from build123d import *

# Parameters (mm, degrees)
SKETCH_3_R = 1.1


with BuildPart() as part:
    # 扫描1: sweep along a path in 草图1
    with BuildLine(Plane.XY) as sweep_1_path:
        Line((2.063476324, 0), (13.736523676, 0))
        ThreePointArc((13.736523676, 0), (15.17265372, 0.608047955), (15.735547828, 2.062469505))
        Line((15.735547828, 2.062469505), (15.343889389, 14.595539539))
        ThreePointArc((15.343889389, 14.595539539), (14.923518493, 15.761017061), (13.897319856, 16.455254701))
        ThreePointArc((13.897319856, 16.455254701), (7.9, 17.3), (1.902680144, 16.455254701))
        ThreePointArc((1.902680144, 16.455254701), (0.876481507, 15.761017061), (0.456110611, 14.595539539))
        Line((0.456110611, 14.595539539), (0.064452172, 2.062469505))
        ThreePointArc((0.064452172, 2.062469505), (0.62734628, 0.608047955), (2.063476324, 0))
    # 草图3 → 扫描1 (sweep)
    with BuildSketch(Plane(origin=(7.6, 0, 0), x_dir=(0, 0, -1), z_dir=(1, 0, 0))):
        Circle(SKETCH_3_R)
    sweep(path=sweep_1_path.line)


solid = part.part
Can you work these out from the model? Positions are in its coordinate system, mm. Give positions to 0.01 mm unless a question says otherwise; leave off trailing zeros. Order: outer loops, then holes, each group sorted by start corner. A loop starts at its lowest first (then second) coordinate and runs counter-clockwise, first axis right, second up. Notation, with made-up numbers: (2.25, 47) - (13.25, 47) arc R22 ccw to (13.25, 69) - close; hole circle Ø9 at (67, 32). An arc over 180 degrees is marked (long way). Write each question's results on one line, items separated by ' | '.
1) Suppose I cut it at A-A, the plane z = 0.25. Write out the boundary of the cut face in (x, y), then the cut area to 3 significant figures.
Final values:
outline: (-1.01, 2.1) arc R3.07 ccw to (2.06, -1.07) - (13.74, -1.07) arc R3.07 ccw to (16.81, 2.1) - (16.41, 14.63) arc R3.07 ccw to (14.19, 17.48) arc R22.78 ccw to (1.61, 17.48) arc R3.07 ccw to (-0.61, 14.63) - close; hole (1.14, 2.03) arc R0.93 ccw to (2.06, 1.07) - (13.74, 1.07) arc R0.93 ccw to (14.66, 2.03) - (14.27, 14.56) arc R0.93 ccw to (13.6, 15.43) arc R20.64 ccw to (2.2, 15.43) arc R0.93 ccw to (1.53, 14.56) - close | area: 129 mm^2
2) Please list where these lines run through material, in increasing order: line 1 along Y through (x, z) = (9.75, 0.4); line 2 along X through (y, z) = (8, -0.7); line 3 along X through (y, z) = (1.75, 0.5). Write a range as [from, to].
Final values:
line 1: y = [-1.02, 1.02], [16.19, 18.25] | line 2: x = [-0.6, 1.1], [14.7, 16.4] | line 3: x = [-0.91, 1.07], [14.73, 16.71]
3) If we mould it in two halves opening along X, with no side actions, what happens to faces 1 (the face through (7.98, 0.33, -1.05)), 2 (the face through (16.51, 8.45, -0.51))? For each: pulls with the +X half, pulls with the -X half, needs draft (parallel to the pull), parting line crosses it, or undercut.
Final values:
face 1: undercut | face 2: undercut
4) I'm going to push flat-ended pins straight in: pin 1 Ø3 at (x, y) = (15, 11) entering from +Z; pin 2 Ø1 at (y, z) = (14, -1) entering from +X. Where does each tip first touch, or does it pass through?
Final values:
pin 1: stops at z = 1.1 | pin 2: stops at x = 16.34
